from build123d import *

# Parameters (mm, degrees)
SKETCH1_R           = 101.6
SKETCH1_R_2         = 63.5
SKETCH1_R_3         = 3.175
BOSS_EXTRUDE1_DEPTH = 139.7
SKETCH5_R           = 101.6
SKETCH5_R_2         = 3.175
SKETCH5_R_3         = 76.2
CUT_EXTRUDE3_DEPTH  = 127


with BuildPart() as part:
    # Sketch1 → Boss-Extrude1 (new body, symmetric)
    with BuildSketch(Plane(origin=(0, 0, 0), x_dir=(1, 0, 0), z_dir=(0, 1, 0))):
        Circle(SKETCH1_R)
        Circle(SKETCH1_R_2, mode=Mode.SUBTRACT)
        with Locations((0, 88.9)):
            Circle(SKETCH1_R_3, mode=Mode.SUBTRACT)
        with Locations((88.9, 0)):
            Circle(SKETCH1_R_3, mode=Mode.SUBTRACT)
        with Locations((44.45, 76.989658396)):
            Circle(SKETCH1_R_3, mode=Mode.SUBTRACT)
        with Locations((76.989658396, 44.45)):
            Circle(SKETCH1_R_3, mode=Mode.SUBTRACT)
        with Locations((76.989658396, -44.45)):
            Circle(SKETCH1_R_3, mode=Mode.SUBTRACT)
        with Locations((44.45, -76.989658396)):
            Circle(SKETCH1_R_3, mode=Mode.SUBTRACT)
        with Locations((0, -88.9)):
            Circle(SKETCH1_R_3, mode=Mode.SUBTRACT)
        with Locations((-44.45, -76.989658396)):
            Circle(SKETCH1_R_3, mode=Mode.SUBTRACT)
        with Locations((-76.989658396, -44.45)):
            Circle(SKETCH1_R_3, mode=Mode.SUBTRACT)
        with Locations((-88.9, 0)):
            Circle(SKETCH1_R_3, mode=Mode.SUBTRACT)
        with Locations((-76.989658396, 44.45)):
            Circle(SKETCH1_R_3, mode=Mode.SUBTRACT)
        with Locations((-44.45, 76.989658396)):
            Circle(SKETCH1_R_3, mode=Mode.SUBTRACT)
    extrude(amount=BOSS_EXTRUDE1_DEPTH, both=True)

    # Sketch5 → Cut-Extrude3 (cut, symmetric)
    with BuildSketch(Plane(origin=(0, 0, 0), x_dir=(1, 0, 0), z_dir=(0, 1, 0))):
        Circle(SKETCH5_R)
        with Locations((-44.45, 76.989658396)):
            Circle(SKETCH5_R_2, mode=Mode.SUBTRACT)
        with Locations((-88.9, 0)):
            Circle(SKETCH5_R_2, mode=Mode.SUBTRACT)
        with Locations((-76.989658396, -44.45)):
            Circle(SKETCH5_R_2, mode=Mode.SUBTRACT)
        with Locations((-44.45, -76.989658396)):
            Circle(SKETCH5_R_2, mode=Mode.SUBTRACT)
        with Locations((0, -88.9)):
            Circle(SKETCH5_R_2, mode=Mode.SUBTRACT)
        with Locations((44.45, -76.989658396)):
            Circle(SKETCH5_R_2, mode=Mode.SUBTRACT)
        with Locations((76.989658396, -44.45)):
            Circle(SKETCH5_R_2, mode=Mode.SUBTRACT)
        with Locations((88.9, 0)):
            Circle(SKETCH5_R_2, mode=Mode.SUBTRACT)
        with Locations((76.989658396, 44.45)):
            Circle(SKETCH5_R_2, mode=Mode.SUBTRACT)
        with Locations((44.45, 76.989658396)):
            Circle(SKETCH5_R_2, mode=Mode.SUBTRACT)
        with Locations((-76.989658396, 44.45)):
            Circle(SKETCH5_R_2, mode=Mode.SUBTRACT)
        with Locations((0, 88.9)):
            Circle(SKETCH5_R_2, mode=Mode.SUBTRACT)
        Circle(SKETCH5_R_3, mode=Mode.SUBTRACT)
    extrude(amount=CUT_EXTRUDE3_DEPTH, both=True, mode=Mode.SUBTRACT)


solid = part.part
Geometry: final body of the model. Coordinates: model frame, mm. A direction names the side the tool comes from. Round coordinates to 2 decimals unless told otherwise and drop trailing zeros. Order: outer loops, then holes, each group sorted by start corner. A loop starts at its lowest first (then second) coordinate and runs counter-clockwise, first axis right, second up. Notation, with made-up numbers: (67, 19.25) -> (115, 19.25) arc R22 cw to (115, 55.25) -> close; hole circle Ø11 at (-22, 25.25). An arc over 180 degrees is marked (long way). Put each result on its own line as item: value. Start each with the question number.
Q1. Line query: probe 1 along Z at (x, y) = (0, 134.75) (3 decimals); probe 2 along X at (y, z) = (42, 0); probe 3 along Z at (x, y) = (-44.45, 130). Output: solid intervals per line, ascending.
Q2. Pull-direction query (X, two-part tool) for faces 1 (the cylindrical face through (74.65, -133.439, -46.596)), 2 (the cylindrical face through (76.6, 133.3, 41.3)), 3 (the flat face through (67, 127, 37)), 4 (the cylindrical face through (-22.025, 133.439, 99.184)); classes: +X half, -X half, draft (parallel to the pull), parting line (faces both ways), or undercut.
Q3. First-contact query: pin 1 (5 mm diameter, centred on y = 3, z = -52.5, fed in from +X); pin 2 (4 mm diameter, centred on x = -88.9, z = 0, fed in from +Y); pin 3 (1.5 mm diameter, centred on y = 93.5, z = 32.5, fed in from -X); pin 4 (1 mm diameter, centred on y = 34, z = 57.5, fed in from +X). Flat tips, straight axial feed; report the tip coordinate or a pass-through.
Q4. Reachability of faces 5 (the cylindrical face through (76.6, -133.4, 41.3)), 6 (the flat face through (67, -127, 37)) from +Z, -Z, +X, -X, +Y, -Y: full face, straight path, thin tool, end or side. Return the list, or none.
Q5. Section A-A on z = -35.5. Return the cut outline in (x, y).
Q6. Section B-B on x = 30. Return the cut outline in (y, z), and give its area (3 significant figures).
Q7. Section C-C on y = -44. Return the cut outline in (x, z).
Ans:
1. probe 1: z = -101.6 to -92.075, -85.725 to -63.5, 63.5 to 85.725, 92.075 to 101.6
1. probe 2: x = -76.2 to -63.5, 63.5 to 76.2
1. probe 3: z = -91.36 to -80.16, -73.81 to -45.35, 45.35 to 73.81, 80.16 to 91.36
2. face 1: undercut
2. face 2: undercut
2. face 3: draft
2. face 4: parting line
3. pin 1: stops at x = 57.5
3. pin 2: passes through
3. pin 3: stops at x = -69.27
3. pin 4: stops at x = 50.57
4. face 5: +Y, -Y
4. face 6: none
5. outline: (-95.2, -139.7) -> (-52.65, -139.7) -> (-52.65, 139.7) -> (-95.2, 139.7) -> (-95.2, 127) -> (-67.43, 127) -> (-67.43, -127) -> (-95.2, -127) -> close; (52.65, -139.7) -> (95.2, -139.7) -> (95.2, -127) -> (67.43, -127) -> (67.43, 127) -> (95.2, 127) -> (95.2, 139.7) -> (52.65, 139.7) -> close
6. outline: (-139.7, -97.07) -> (-127, -97.07) -> (-127, -70.05) -> (127, -70.05) -> (127, -97.07) -> (139.7, -97.07) -> (139.7, -55.97) -> (-139.7, -55.97) -> close; (-139.7, 55.97) -> (139.7, 55.97) -> (139.7, 97.07) -> (127, 97.07) -> (127, 70.05) -> (-127, 70.05) -> (-127, 97.07) -> (-139.7, 97.07) -> close
6. area: 9,240 mm2
7. outline: circle Ø152.4 at (0, 0); hole circle Ø127 at (0, 0)
